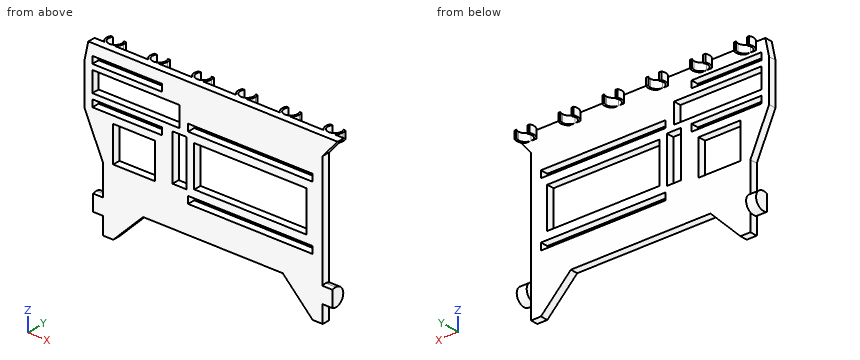
from build123d import *

# Parameters (mm, degrees)
SKETCH1_W            = 88
SKETCH1_H            = 65
SKETCH1_W_2          = 7.5
SKETCH1_H_2          = 33
BOSS_EXTRUDE1_DEPTH  = 3
BOSS_EXTRUDE8_DEPTH  = 4
CUT_EXTRUDE18_DEPTH  = 61.971304726
SKETCH8_W            = 16
SKETCH8_H            = 45
SKETCH8_W_2          = 2.75
SKETCH8_H_2          = 50
SKETCH8_W_3          = 18.1
SKETCH8_H_3          = 4.25
SKETCH8_H_4          = 1.5
CUT_EXTRUDE19_DEPTH  = 64.044492712
SKETCH10_W           = 16.75
SKETCH10_H           = 14
CUT_EXTRUDE21_DEPTH  = 61.971304726
BOSS_EXTRUDE10_DEPTH = 3
BOSS_EXTRUDE9_START  = -3
BOSS_EXTRUDE9_DEPTH  = 3
SKETCH16_W           = 35
SKETCH16_H           = 8
CUT_EXTRUDE22_DEPTH  = 3
SKETCH17_W           = 28
SKETCH17_H           = 2.75
CUT_EXTRUDE23_DEPTH  = 3
CUT_EXTRUDE24_DEPTH  = 3


# Read off the part's stored shape, not the designer's step: Boss-Extrude9
with BuildPart() as part:
    # Sketch1 → Boss-Extrude1 (new body)
    with BuildSketch(Plane(origin=(0, 0, 0), x_dir=(1, 0, 0), z_dir=(0, 1, 0))):
        Rectangle(SKETCH1_W, SKETCH1_H)
        with Locations((-47.75, -9)):
            Rectangle(SKETCH1_W_2, SKETCH1_H_2)
        with Locations((47.75, -9)):
            Rectangle(SKETCH1_W_2, SKETCH1_H_2)
    extrude(amount=BOSS_EXTRUDE1_DEPTH)

    # Sketch2 → Boss-Extrude8 (add)
    with BuildSketch(Plane.ZY.offset(44)):
        with BuildLine():
            ThreePointArc((-19, 1.5), (-23.268774411, 4.914525722), (-25.66227766, 0))
            Line((-25.66227766, 0), (-19.33772234, 0))
            ThreePointArc((-19.33772234, 0), (-19.085474278, 0.731225589), (-19, 1.5))
        make_face()
    boss_extrude8 = extrude(amount=BOSS_EXTRUDE8_DEPTH)

    # Sketch7 → Cut-Extrude18 (cut, through all)
    with BuildSketch(Plane(origin=(0, 3, 0), x_dir=(1, 0, 0), z_dir=(0, 1, 0))):
        Polygon((-40, 32.5), (-28, 20.5), (0, 20.5), (0, 32.5), align=None)
    cut_extrude18 = extrude(amount=-CUT_EXTRUDE18_DEPTH, mode=Mode.SUBTRACT)

    # Mirror4: Cut-Extrude18 across plane
    add(cut_extrude18.mirror(Plane(origin=(0, 0, 0), x_dir=(0, 0, 1), z_dir=(1, 0, 0))), mode=Mode.SUBTRACT)

    # Mirror5: Boss-Extrude8 across plane
    add(boss_extrude8.mirror(Plane(origin=(0, 0, 0), x_dir=(0, 0, 1), z_dir=(1, 0, 0))))

    # Sketch8 → Cut-Extrude19 (cut, through all)
    with BuildSketch(Plane(origin=(1.47526487, 3, -1.547457662), x_dir=(0, 0, -1), z_dir=(0, 1, 0))):
        with Locations((-5.672457662, -13.52473513)):
            Rectangle(SKETCH8_W, SKETCH8_H)
        with Locations((6.802542338, -13.521195307)):
            Rectangle(SKETCH8_W_2, SKETCH8_H_2)
        with Locations((-18.147457662, -13.521195307)):
            Rectangle(SKETCH8_W_2, SKETCH8_H_2)
        with Locations((-5.672457662, 15.60026487)):
            Rectangle(SKETCH8_W_3, SKETCH8_H_3)
        with Locations((-5.672457662, 12.72526487)):
            Rectangle(SKETCH8_W_3, SKETCH8_H_4)
    extrude(amount=-CUT_EXTRUDE19_DEPTH, mode=Mode.SUBTRACT)

    # Sketch10 → Cut-Extrude21 (cut, through all)
    with BuildSketch(Plane(origin=(0, 3, 0), x_dir=(1, 0, 0), z_dir=(0, 1, 0))):
        with Locations((-31.625, -0.5)):
            Rectangle(SKETCH10_W, SKETCH10_H)
    extrude(amount=-CUT_EXTRUDE21_DEPTH, mode=Mode.SUBTRACT)

    # Sketch15 → Boss-Extrude10 (add)
    with BuildSketch(Plane.XY.offset(32.5)):
        with BuildLine():
            Line((-46.184605227, 7.15), (-47.05122926, 7.15))
            ThreePointArc((-47.05122926, 7.15), (-46.886173938, 3.852779924), (-44, 2.25))
            Line((-44, 2.25), (-44, 3))
            ThreePointArc((-44, 3), (-46.344941364, 4.41559731), (-46.184605227, 7.15))
        make_face()
        with BuildLine():
            ThreePointArc((-40.6, 5.65), (-40.688340334, 6.42000666), (-40.94877074, 7.15))
            Line((-40.94877074, 7.15), (-41.815394773, 7.15))
            ThreePointArc((-41.815394773, 7.15), (-41.469021548, 6.435269427), (-41.35, 5.65))
            ThreePointArc((-41.35, 5.65), (-42.12616703, 3.77616703), (-44, 3))
            Line((-44, 3), (-41.86985916, 3))
            ThreePointArc((-41.86985916, 3), (-40.933855935, 4.180727877), (-40.6, 5.65))
        make_face()
        with BuildLine():
            ThreePointArc((-29.45122926, 7.15), (-29.719227927, 4.913300625), (-28.53014084, 3))
            Line((-28.53014084, 3), (-26.4, 3))
            ThreePointArc((-26.4, 3), (-28.744941364, 4.41559731), (-28.584605227, 7.15))
            Line((-28.584605227, 7.15), (-29.45122926, 7.15))
        make_face()
        with BuildLine():
            Line((-26.4, 3), (-24.26985916, 3))
            ThreePointArc((-24.26985916, 3), (-23.333855935, 4.180727877), (-23, 5.65))
            ThreePointArc((-23, 5.65), (-23.088340334, 6.42000666), (-23.34877074, 7.15))
            Line((-23.34877074, 7.15), (-24.215394773, 7.15))
            ThreePointArc((-24.215394773, 7.15), (-23.869021548, 6.435269427), (-23.75, 5.65))
            ThreePointArc((-23.75, 5.65), (-24.52616703, 3.77616703), (-26.4, 3))
        make_face()
        with BuildLine():
            Line((-8.8, 3), (-6.66985916, 3))
            ThreePointArc((-6.66985916, 3), (-5.733855935, 4.180727877), (-5.4, 5.65))
            ThreePointArc((-5.4, 5.65), (-5.488340334, 6.42000666), (-5.74877074, 7.15))
            Line((-5.74877074, 7.15), (-6.615394773, 7.15))
            ThreePointArc((-6.615394773, 7.15), (-6.269021548, 6.435269427), (-6.15, 5.65))
            ThreePointArc((-6.15, 5.65), (-6.92616703, 3.77616703), (-8.8, 3))
        make_face()
        with BuildLine():
            ThreePointArc((-11.85122926, 7.15), (-12.119227927, 4.913300625), (-10.93014084, 3))
            Line((-10.93014084, 3), (-8.8, 3))
            ThreePointArc((-8.8, 3), (-11.144941364, 4.41559731), (-10.984605227, 7.15))
            Line((-10.984605227, 7.15), (-11.85122926, 7.15))
        make_face()
        with BuildLine():
            Line((8.800000027, 3), (10.93014084, 3))
            ThreePointArc((10.93014084, 3), (11.866144065, 4.180727877), (12.2, 5.65))
            ThreePointArc((12.2, 5.65), (12.111659666, 6.42000666), (11.85122926, 7.15))
            Line((11.85122926, 7.15), (10.984605227, 7.15))
            ThreePointArc((10.984605227, 7.15), (11.330978452, 6.435269427), (11.45, 5.65))
            ThreePointArc((11.45, 5.65), (10.67383298, 3.77616704), (8.800000027, 3))
        make_face()
        with BuildLine():
            ThreePointArc((5.74877074, 7.15), (5.480772073, 4.913300625), (6.66985916, 3))
            Line((6.66985916, 3), (8.800000027, 3))
            ThreePointArc((8.800000027, 3), (6.455058643, 4.415597298), (6.615394773, 7.15))
            Line((6.615394773, 7.15), (5.74877074, 7.15))
        make_face()
        with BuildLine():
            Line((26.4, 3), (28.53014084, 3))
            ThreePointArc((28.53014084, 3), (29.466144065, 4.180727877), (29.8, 5.65))
            ThreePointArc((29.8, 5.65), (29.711659666, 6.42000666), (29.45122926, 7.15))
            Line((29.45122926, 7.15), (28.584605227, 7.15))
            ThreePointArc((28.584605227, 7.15), (28.930978452, 6.435269427), (29.05, 5.65))
            ThreePointArc((29.05, 5.65), (28.27383297, 3.77616703), (26.4, 3))
        make_face()
        with BuildLine():
            ThreePointArc((23.34877074, 7.15), (23.080772073, 4.913300625), (24.26985916, 3))
            Line((24.26985916, 3), (26.4, 3))
            ThreePointArc((26.4, 3), (24.055058636, 4.41559731), (24.215394773, 7.15))
            Line((24.215394773, 7.15), (23.34877074, 7.15))
        make_face()
        with BuildLine():
            ThreePointArc((40.94877074, 7.15), (40.680772073, 4.913300625), (41.86985916, 3))
            Line((41.86985916, 3), (44, 3))
            ThreePointArc((44, 3), (41.655058636, 4.41559731), (41.815394773, 7.15))
            Line((41.815394773, 7.15), (40.94877074, 7.15))
        make_face()
        with BuildLine():
            ThreePointArc((47.4, 5.65), (47.311659666, 6.42000666), (47.05122926, 7.15))
            Line((47.05122926, 7.15), (46.184605227, 7.15))
            ThreePointArc((46.184605227, 7.15), (46.530978452, 6.435269427), (46.65, 5.65))
            ThreePointArc((46.65, 5.65), (45.87383297, 3.77616703), (44, 3))
            Line((44, 3), (44, 2.25))
            ThreePointArc((44, 2.25), (46.404163056, 3.245836944), (47.4, 5.65))
        make_face()
    extrude(amount=-BOSS_EXTRUDE10_DEPTH)

    # Boss-Extrude9 outline → Boss-Extrude9 (add)
    with BuildSketch(Plane(origin=(0, 3, 0), x_dir=(1, 0, 0), z_dir=(0, 1, 0)).offset(BOSS_EXTRUDE9_START)):
        Polygon((-50, -32.5), (-44, -32.5), (-44, -29.5), (-44, -25.5), (-51.5, -25.5), align=None)
        Polygon((44, -32.5), (50, -32.5), (51.5, -25.5), (44, -25.5), (44, -29.5), align=None)
    extrude(amount=BOSS_EXTRUDE9_DEPTH)

    # Sketch16 → Cut-Extrude22 (cut)
    with BuildSketch(Plane(origin=(0, 3, 0), x_dir=(1, 0, 0), z_dir=(0, 1, 0))):
        with Locations((-30.875, -19.225)):
            Rectangle(SKETCH16_W, SKETCH16_H)
    extrude(amount=-CUT_EXTRUDE22_DEPTH, mode=Mode.SUBTRACT)

    # Sketch17 → Cut-Extrude23 (cut)
    with BuildSketch(Plane(origin=(0, 3, 0), x_dir=(1, 0, 0), z_dir=(0, 1, 0))):
        with Locations((-34.375, -11.725)):
            Rectangle(SKETCH17_W, SKETCH17_H)
        with Locations((-34.375, -26.725)):
            Rectangle(SKETCH17_W, SKETCH17_H)
    extrude(amount=-CUT_EXTRUDE23_DEPTH, mode=Mode.SUBTRACT)

    # Sketch19 → Cut-Extrude24 (cut)
    with BuildSketch(Plane(origin=(0, 3, 0), x_dir=(1, 0, 0), z_dir=(0, 1, 0))):
        Polygon((50, -32.5), (51.5, -25.5), (51.5, 7.5), (44, 7.5), (44, -25.5), align=None)
        Polygon((-51.5, -9), (-44, 7.5), (-51.5, 7.5), align=None)
    extrude(amount=-CUT_EXTRUDE24_DEPTH, mode=Mode.SUBTRACT)


solid = part.part
Design review of the part built by this model. Coordinates are the model's own, in mm. Coordinates: 2 decimals unless noted, no trailing zeros. Order: outer loops, then holes, each group sorted by start corner. A loop starts at its lowest first (then second) coordinate and runs counter-clockwise, first axis right, second up. Notation, with made-up numbers: (-36.75, 14) -> (-19.75, 14) arc R20 ccw to (-19.75, 51) -> close; hole circle Ø6 at (56.5, 23). An arc over 180 degrees is marked (long way). One line per item, written item: value.
1) Clearance check with flat-ended pins moving along their axes: P1, Ø1, axis at x = 3.5, z = 15.5, coming from the +Y side; P2, Ø2, axis at y = 2, z = -5, coming from the +X side; P3, Ø3.5, axis at x = -46, y = 6, coming from the -Z side. State where each tip first meets the part, or that it passes through.
Output values:
P1: stops at y = 3
P2: stops at x = 44
P3: stops at z = -24.67
2) We need section D-D, the plane z = 2. Give the boundary of the cut face in (x, y).
Output values:
outline: (-48.32, 0) -> (-40, 0) -> (-40, 3) -> (-48.32, 3) -> close; (-23.25, 0) -> (-16.25, 0) -> (-16.25, 3) -> (-23.25, 3) -> close; (-10.5, 0) -> (-7.5, 0) -> (-7.5, 3) -> (-10.5, 3) -> close; (37.5, 0) -> (44, 0) -> (44, 3) -> (37.5, 3) -> close
3) We need section B-B, the plane x = 3.5. Give the boundary of the cut face in (y, z) (3 decimals).
Output values:
outline: (0, -20.5) -> (3, -20.5) -> (3, -9.725) -> (0, -9.725) -> close; (0, -6.975) -> (3, -6.975) -> (3, -3.875) -> (0, -3.875) -> close; (0, 12.125) -> (3, 12.125) -> (3, 15.225) -> (0, 15.225) -> close; (0, 17.975) -> (3, 17.975) -> (3, 32.5) -> (0, 32.5) -> close
4) To check wall thickness, follow probe 1 along Z at (x, y) = (16.5, 2.5) (3 decimals); probe 2 along Z at (x, y) = (-14.5, 1) (3 decimals); probe 3 along X at (y, z) = (2, 9). State the ranges of each line that lie inside material, in increasing order. Write a range as [from, to].
Output values:
probe 1: z = [-20.5, -9.725], [-6.975, -3.875], [12.125, 15.225], [17.975, 32.5]
probe 2: z = [-20.5, -4.925], [13.175, 15.225], [23.225, 32.5]
probe 3: x = [-51.5, -16.25], [-10.5, -7.5], [37.5, 44]
5) We need section A-A, the plane z = -22.5. Give the boundary of the cut face in (x, y), then the cut area to 3 significant figures.
Output values:
outline: (-48, 0) -> (-30, 0) -> (-30, 3) -> (-44, 3) -> (-44, 5) -> (-48, 5) -> close; (30, 0) -> (48, 0) -> (48, 5) -> (44, 5) -> (44, 3) -> (30, 3) -> close
area: 124 mm2
6) We need section C-C, the plane z = 17. Give the boundary of the cut face in (x, y) (3 decimals).
Output values:
outline: (-51.5, 0) -> (-48.375, 0) -> (-48.375, 3) -> (-51.5, 3) -> close; (-13.375, 0) -> (-10.004, 0) -> (-10.004, 3) -> (-13.375, 3) -> close; (39.996, 0) -> (44, 0) -> (44, 3) -> (39.996, 3) -> close
